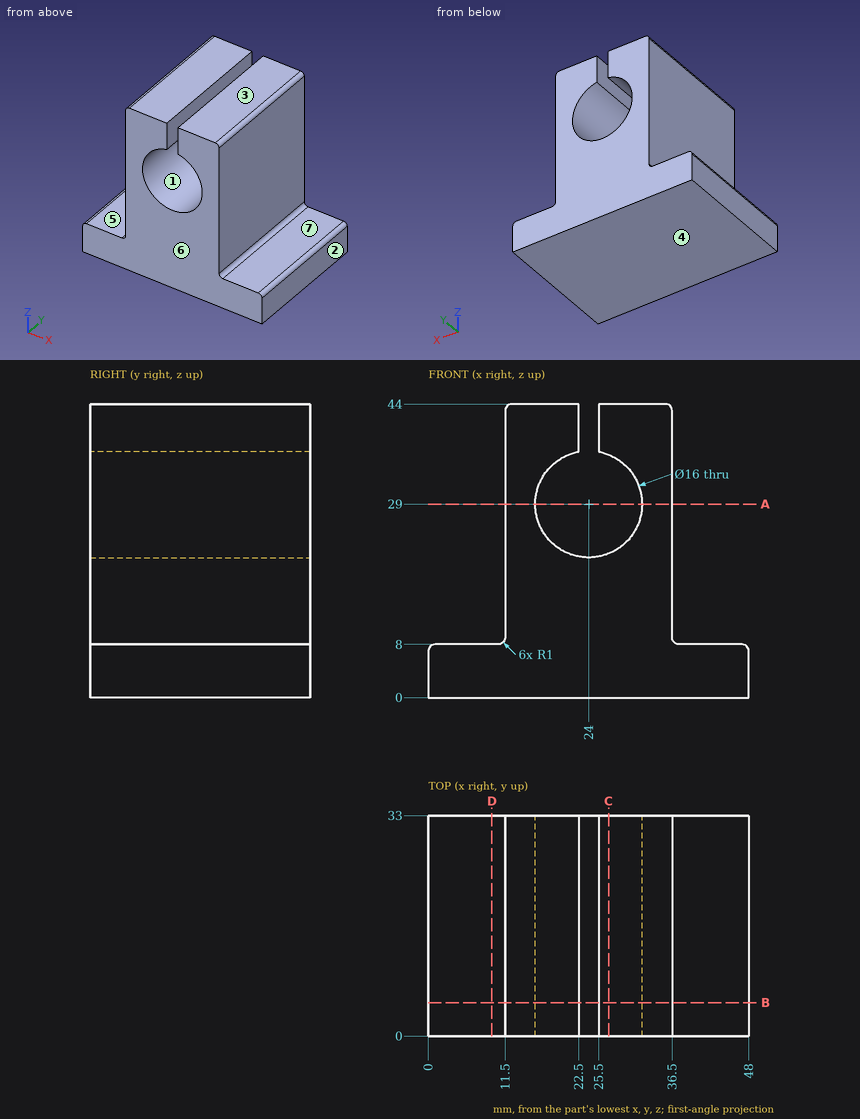
Study the drawing (mm; zero at the part's minimum x, y, z) and answer. A direction names the side the tool comes from. Coordinates: 2 decimals unless noted, no trailing zeros. Write each loop counter-clockwise with the first axis right and the second up, starting at its lowest first coordinate (ties: lowest second). Pieces come first, ordered by that corner, then holes.
Q1. A cutting plane is placed at A-A, the plane z = 29. Give the vertices of the cut face in (x, y), then the cut area to 3 significant figures.
Q2. Which of the six approach directions +Z, -Z, +X, -X, +Y, -Y give full straight-line access (tool end or side, diameter ignored) to the marked faces 5, 6 and 7?
Q3. Find the intervals of material crossed by line 1 (Z direction, x = 24, y = 17.5); line 2 (X direction, y = 13, z = 29); line 3 (Z direction, x = 8.5, y = 2), in increasing order.
Q4. A cutting plane is placed at C-C, the plane x = 27. Give the vertices of the cut face in (y, z).
Q5. Determine the mould class of the marked faces 1, 2, 3 and 4 for opening direction Z: released by +Z, released by -Z, zero draft, split by the parting line, or undercut.
Q6. Each of these flat-tipped pins is pushed along its axis until it touches: pin 1 Ø1.5 at (y, z) = (6.5, 8) entering from -X; pin 2 Ø2 at (y, z) = (20.5, 25) entering from +X; pin 3 Ø7.5 at (x, y) = (5.5, 9.5) entering from +Z. Where does it stop, or does it pass through?
Q7. A cutting plane is placed at B-B, the plane y = 5. Give the vertices of the cut face in (x, z).
Q8. A cutting plane is placed at D-D, the plane x = 9.5. Give the vertices of the cut face in (y, z).
Findings below:
1. outline: (11.5, 0) - (16, 0) - (16, 33) - (11.5, 33) - close; (32, 0) - (36.5, 0) - (36.5, 33) - (32, 33) - close
1. area: 297 mm2
2. face 5: +Z, -X, +Y, -Y
2. face 6: +Z, -Z, +X, -X, -Y
2. face 7: +Z, +X, +Y, -Y
3. line 1: z = 0 to 21
3. line 2: x = 11.5 to 16, 32 to 36.5
3. line 3: z = 0 to 8
4. outline: (0, 0) - (33, 0) - (33, 21.58) - (0, 21.58) - close; (0, 36.42) - (33, 36.42) - (33, 44) - (0, 44) - close
5. face 1: undercut
5. face 2: zero draft
5. face 3: released by +Z
5. face 4: released by -Z
6. pin 1: stops at x = 0.03
6. pin 2: stops at x = 36.5
6. pin 3: stops at z = 8
7. outline: (0, 0) - (48, 0) - (48, 7) arc R1 ccw to (47, 8) - (37.5, 8) arc R1 cw to (36.5, 9) - (36.5, 43) arc R1 ccw to (35.5, 44) - (25.5, 44) - (25.5, 36.86) arc R8 cw (long way) to (22.5, 36.86) - (22.5, 44) - (12.5, 44) arc R1 ccw to (11.5, 43) - (11.5, 9) arc R1 cw to (10.5, 8) - (1, 8) arc R1 ccw to (0, 7) - close
8. outline: (0, 0) - (33, 0) - (33, 8) - (0, 8) - close
